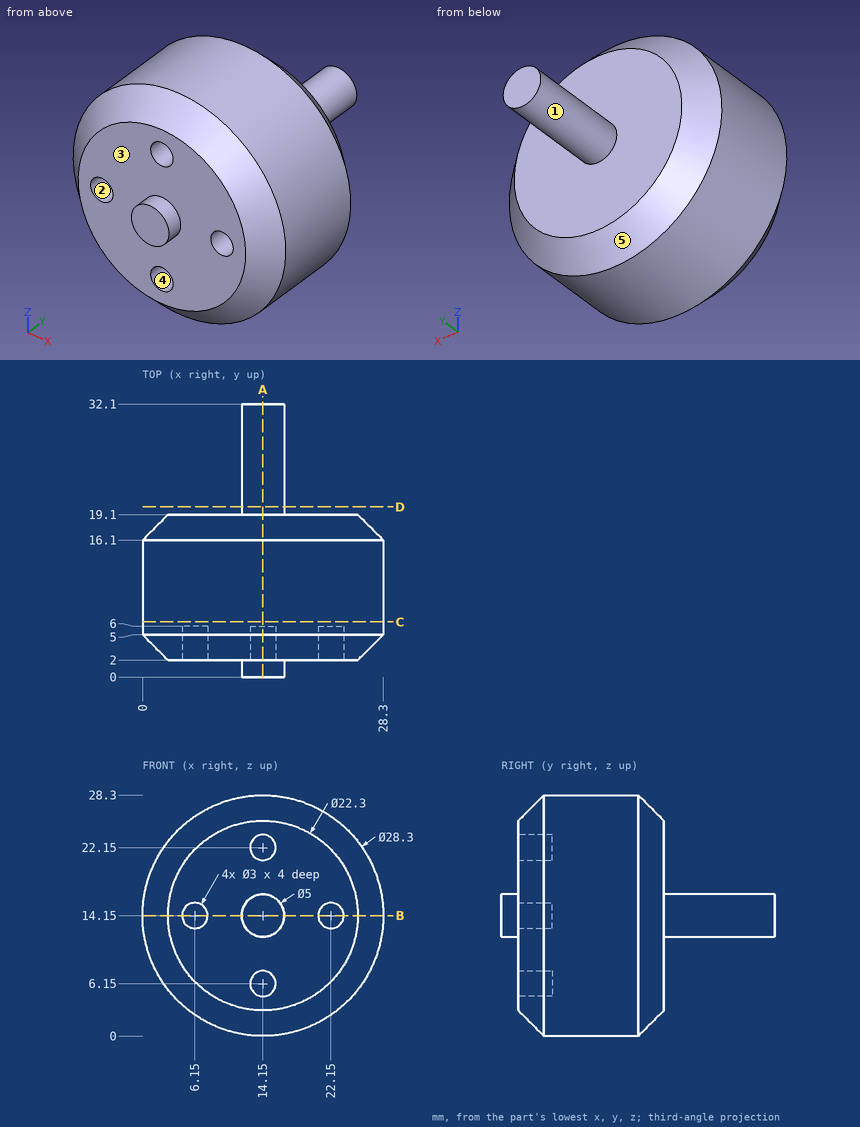
Part print with two shaded views. Sizes in mm from the minimum x, y, z corner. A direction names the side the tool comes from. Give positions to 0.01 mm unless a question says otherwise; leave off trailing zeros. Order: outer loops, then holes, each group sorted by start corner. A loop starts at its lowest first (then second) coordinate and runs counter-clockwise, first axis right, second up. Notation, with made-up numbers: M 39,11.25 L 95,11.25 A33 cw 95,47.25 Z; hole C 13,37 d3. An arc over 180 degrees is marked long. Write item = value, one per line.
Q1. Two-plate mould, pull along X, no slides. Class the marked faces 1, 2 and 3: pulls with the +X half, pulls with the -X half, needs draft (parallel to the pull), parting line crosses it, or undercut.
Derived:
face_1 = parting line crosses it
face_2 = undercut
face_3 = needs draft
Q2. Cut at D-D, the plane y = 20. List the corners of the cut face in (x, z), then the cut area to 3 significant figures.
Derived:
outline = C 14.15,14.15 d5
area = 19.6 mm2
Q3. Cut at C-C, the plane y = 6.5. List the corners of the cut face in (x, z).
Derived:
outline = C 14.15,14.15 d28.3
Q4. Drill centre lines: line 1 (X direction, y = 3.9, z = 14.15); line 2 (Z direction, x = 22.15, y = 2.8); line 3 (X direction, y = 4.85, z = 22.15). Where is each one in solid material? Low to high. Write a range as [from, to].
Derived:
line_1 = [1.1, 4.65], [7.65, 20.65], [23.65, 27.2]
line_2 = [5.27, 12.65], [15.65, 23.03]
line_3 = [2.66, 12.65], [15.65, 25.64]
Q5. Flat gauge pins, fed straight in: pin 1 (4 mm diameter, centred on x = 22.15, z = 14.15, fed in from -Y); pin 2 (5 mm diameter, centred on y = 16.5, z = 5.5, fed in from -X); pin 3 (10 mm diameter, centred on x = 23.5, y = 9.5, fed in from +Z). Where does each tip first touch, or does it go through?
Derived:
pin_1 = 2
pin_2 = 1.42
pin_3 = 27.61
Q6. Tool access for the marked faces 4 and 5: list every direction of +Z, -Z, +X, -X, +Y, -Y with a clear straight run to the whole face (end or side of a thin tool).
Derived:
face_4 = -Y
face_5 = +Y
Q7. Cut at A-A, the plane x = 14.15. List the corners of the cut face in (y, z), then the cut area to 3 significant figures.
Derived:
outline = M 0,11.65 L 2,11.65 L 2,7.65 L 6,7.65 L 6,4.65 L 2,4.65 L 2,3 L 5,0 L 16.1,0 L 19.1,3 L 19.1,11.65 L 32.1,11.65 L 32.1,16.65 L 19.1,16.65 L 19.1,25.3 L 16.1,28.3 L 5,28.3 L 2,25.3 L 2,23.65 L 6,23.65 L 6,20.65 L 2,20.65 L 2,16.65 L 0,16.65 Z
area = 517 mm2
Q8. Cut at B-B, the plane z = 14.15. List the corners of the cut face in (x, y), then the cut area to 3 significant figures.
Derived:
outline = M 0,5 L 3,2 L 4.65,2 L 4.65,6 L 7.65,6 L 7.65,2 L 11.65,2 L 11.65,0 L 16.65,0 L 16.65,2 L 20.65,2 L 20.65,6 L 23.65,6 L 23.65,2 L 25.3,2 L 28.3,5 L 28.3,16.1 L 25.3,19.1 L 16.65,19.1 L 16.65,32.1 L 11.65,32.1 L 11.65,19.1 L 3,19.1 L 0,16.1 Z
area = 517 mm2
